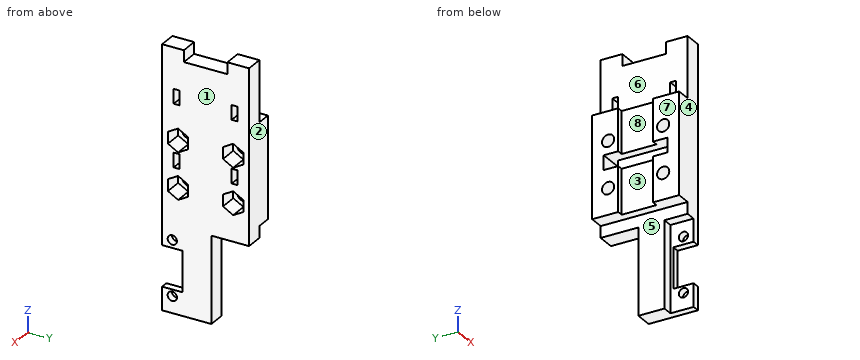
```python
from build123d import *

# Parameters (mm, degrees)
BOSS_EXTRUDE1_DEPTH = 30
CUT_EXTRUDE1_REACH  = 53.981
SKETCH2_R           = 2.1
CUT_EXTRUDE2_DEPTH  = 6
SKETCH4_W           = 5
SKETCH4_H           = 2
CUT_EXTRUDE3_DEPTH  = 52.980765673
SKETCH5_W           = 5
SKETCH5_H           = 18
CUT_EXTRUDE4_DEPTH  = 5
SKETCH6_W           = 4
SKETCH6_H           = 15
CUT_EXTRUDE5_DEPTH  = 52.15662225
BOSS_EXTRUDE2_DEPTH = 5
SKETCH7_W           = 2
SKETCH7_H           = 12
CUT_EXTRUDE6_DEPTH  = 51.418250664
LPATTERN1_COUNT     = 2
LPATTERN1_PITCH     = 16
BOSS_EXTRUDE3_DEPTH = 2.5
SKETCH10_W          = 29.8
SKETCH10_H          = 9
BOSS_EXTRUDE4_DEPTH = 3.5
SKETCH11_R          = 1.6
CUT_EXTRUDE7_DEPTH  = 59.330438023


with BuildPart() as part:
    # Sketch1 → Boss-Extrude1 (new body)
    with BuildSketch(Plane(origin=(0, 0, 0), x_dir=(1, 0, 0), z_dir=(0, 1, 0))):
        Polygon((0, 0), (5, 0), (5, 19), (11, 19), (11, -41), (5, -41), (5, -20), (0, -20), align=None)
    extrude(amount=BOSS_EXTRUDE1_DEPTH)

    # Sketch2 → Cut-Extrude1 (cut, up to next)
    with BuildSketch(Plane(origin=(11, 0, 0), x_dir=(0, 0, -1), z_dir=(1, 0, 0)), mode=Mode.PRIVATE) as cut_extrude1_sk1:
        with Locations((-10, 24.5)):
            Circle(SKETCH2_R)
    cut_extrude1_tool1 = extrude(cut_extrude1_sk1.sketch, amount=-CUT_EXTRUDE1_REACH, mode=Mode.PRIVATE) & part.part
    # Sketch2 → Cut-Extrude1 (cut, up to next)
    with BuildSketch(Plane(origin=(11, 0, 0), x_dir=(0, 0, -1), z_dir=(1, 0, 0)), mode=Mode.PRIVATE) as cut_extrude1_sk2:
        with Locations((-10, 5.5)):
            Circle(SKETCH2_R)
    cut_extrude1_tool2 = extrude(cut_extrude1_sk2.sketch, amount=-CUT_EXTRUDE1_REACH, mode=Mode.PRIVATE) & part.part
    cut_extrude1_1 = cut_extrude1_tool1.solids().sort_by_distance((11, 24.5, 10))[0]
    add(cut_extrude1_1, mode=Mode.SUBTRACT)
    cut_extrude1_2 = cut_extrude1_tool2.solids().sort_by_distance((11, 5.5, 10))[0]
    add(cut_extrude1_2, mode=Mode.SUBTRACT)
    cut_extrude1 = cut_extrude1_1 + cut_extrude1_2  # Cut-Extrude1 as one shape, for the pattern or mirror that repeats it

    # Sketch3 → Cut-Extrude2 (cut)
    with BuildSketch(Plane(origin=(11, 0, 0), x_dir=(0, 0, -1), z_dir=(1, 0, 0))):
        Polygon((-14.041451884, 24.5), (-12.020725942, 21), (-7.979274058, 21), (-5.958548116, 24.5), (-7.979274058, 28), (-12.020725942, 28), align=None)
        Polygon((-14.041451884, 5.5), (-12.020725942, 2), (-7.979274058, 2), (-5.958548116, 5.5), (-7.979274058, 9), (-12.020725942, 9), align=None)
    cut_extrude2 = extrude(amount=-CUT_EXTRUDE2_DEPTH, mode=Mode.SUBTRACT)

    # Sketch4 → Cut-Extrude3 (cut, through all)
    with BuildSketch(Plane(origin=(11, 0, 0), x_dir=(0, 0, -1), z_dir=(1, 0, 0))):
        with Locations((-24.5, 25)):
            Rectangle(SKETCH4_W, SKETCH4_H)
        with Locations((-24.5, 5)):
            Rectangle(SKETCH4_W, SKETCH4_H)
        with Locations((-3, 25)):
            Rectangle(SKETCH4_W, SKETCH4_H)
        with Locations((-3, 5)):
            Rectangle(SKETCH4_W, SKETCH4_H)
    extrude(amount=-CUT_EXTRUDE3_DEPTH, mode=Mode.SUBTRACT)

    # Sketch5 → Cut-Extrude4 (cut)
    with BuildSketch(Plane.ZY):
        with Locations((3, 15)):
            Rectangle(SKETCH5_W, SKETCH5_H)
    extrude(amount=-CUT_EXTRUDE4_DEPTH, mode=Mode.SUBTRACT)

    # Sketch6 → Cut-Extrude5 (cut, through all)
    with BuildSketch(Plane.ZY.offset(-5)):
        with Locations((39, 15)):
            Rectangle(SKETCH6_W, SKETCH6_H)
    extrude(amount=-CUT_EXTRUDE5_DEPTH, mode=Mode.SUBTRACT)

    # Sketch8 → Boss-Extrude2 (add)
    with BuildSketch(Plane.ZY.offset(-5)):
        Polygon((0, 30), (0, 14.791308029), (0, 0), (-15, 0), (-15, 30), align=None)
    extrude(amount=BOSS_EXTRUDE2_DEPTH)

    # Sketch7 → Cut-Extrude6 (cut, through all)
    with BuildSketch(Plane.XY.offset(20)):
        with Locations((1, 15)):
            Rectangle(SKETCH7_W, SKETCH7_H)
    extrude(amount=-CUT_EXTRUDE6_DEPTH, mode=Mode.SUBTRACT)

    # LPattern1: Cut-Extrude1, Cut-Extrude2 ×2
    with Locations(*[(0, 0, -i * LPATTERN1_PITCH) for i in range(1, LPATTERN1_COUNT)]):
        add(cut_extrude1, mode=Mode.SUBTRACT)
        add(cut_extrude2, mode=Mode.SUBTRACT)

    # Sketch9 → Boss-Extrude3 (add)
    with BuildSketch(Plane(origin=(11, 0, 0), x_dir=(0, 0, -1), z_dir=(1, 0, 0))):
        Polygon((19, 0), (26.8, 0), (26.8, 7), (40.8, 7), (40.8, 0), (48.8, 0), (48.8, 17), (19, 17), align=None)
    extrude(amount=-BOSS_EXTRUDE3_DEPTH)

    # Sketch10 → Boss-Extrude4 (add)
    with BuildSketch(Plane.ZY.offset(-8.5)):
        with Locations((-33.9, 12.5)):
            Rectangle(SKETCH10_W, SKETCH10_H)
    extrude(amount=BOSS_EXTRUDE4_DEPTH)

    # Sketch11 → Cut-Extrude7 (cut, through all)
    with BuildSketch(Plane(origin=(11, 0, 0), x_dir=(0, 0, -1), z_dir=(1, 0, 0))):
        with Locations((43.1, 3.5)):
            Circle(SKETCH11_R)
        with Locations((24.1, 3.5)):
            Circle(SKETCH11_R)
    extrude(amount=-CUT_EXTRUDE7_DEPTH, mode=Mode.SUBTRACT)


solid = part.part
```
Geometry: final body of the model. Coordinates: model frame, mm. Face numbers are marked on the shaded views. A direction names the side the tool comes from. Round coordinates to 2 decimals unless told otherwise and drop trailing zeros. Write each loop counter-clockwise with the first axis right and the second up, starting at its lowest first coordinate (ties: lowest second). Pieces come first, ordered by that corner, then holes. Notation, with made-up numbers: M 44.5,25 L 62.5,25 A29 cw 62.5,62 Z; hole C -9,-10 d7. An arc over 180 degrees is marked long. Answer in a Markdown table with one row per item. Add a question column.
(1) Cut plane C-C, the plane y = 14.25. Return the cut outline in (x, z), then the cut area to 3 significant figures.
(2) Draft query along Y for the marked faces 1, 2 and 3. Return one class per face: pulls with the +Y half, pulls with the -Y half, needs draft (parallel to the pull), parting line crosses it, or undercut.
(3) Cut plane B-B, the plane z = -43.1. Return the cut outline in (x, y).
(4) Cut plane D-D, the plane z = -6. Return the cut outline in (x, y), then the cut area to 3 significant figures.
(5) Reachability of the marked faces 4, 5, 6, 7 and 8 from +Z, -Z, +X, -X, +Y, -Y: full face, straight path, thin tool, end or side. Return the list, or none.
(6) Cut plane A-A, the plane z = 26. Return the cut outline in (x, y).
(7) Ray query, L1, parallel to Z at x = 3.75, y = 25; L2, parallel to Y at x = 1.15, z = -6; L3, parallel to Y at x = 3.35, z = -6. Return the intervals inside material, ascending.
(8) Contact query for flat-ended pins moving along their axis: pin 1 (5.5 mm diameter, centred on y = 5.5, z = 10, fed in from +X); pin 2 (2 mm diameter, centred on x = 7, y = 5, fed in from -Z); pin 3 (5 mm diameter, centred on y = 13.5, z = -29.5, fed in from -X). Output: stop coordinate, or through.
Established:
| question | item | result |
|---|---|---|
| 1 | outline | M 2,-15 L 5,-15 L 5,-48.8 L 11,-48.8 L 11,37 L 5,37 L 5,20 L 2,20 L 2,5.5 L 5,5.5 L 5,0.5 L 2,0.5 Z |
| 1 | area | 605 mm² |
| 2 | face 1 | needs draft |
| 2 | face 2 | pulls with the +Y half |
| 2 | face 3 | undercut |
| 3 | outline | M 5,8 L 8.5,8 L 8.5,5.1 L 11,5.1 L 11,17 L 5,17 Z; M 8.5,0 L 11,0 L 11,1.9 L 8.5,1.9 Z |
| 4 | outline | M 0,0 L 11,0 L 11,2 L 5,2 L 5,3.4 L 0,3.4 Z; M 0,7.6 L 5,7.6 L 5,9 L 11,9 L 11,21 L 5,21 L 5,22.4 L 0,22.4 L 0,21 L 2,21 L 2,9 L 0,9 Z; M 0,26.6 L 5,26.6 L 5,28 L 11,28 L 11,30 L 0,30 Z |
| 4 | area | 180 mm² |
| 5 | face 4 | +Z, -Z, +X, -X, -Y |
| 5 | face 5 | -Z, -X, +Y, -Y |
| 5 | face 6 | +Z, -X, +Y, -Y |
| 5 | face 7 | +Z, -Z, -X, +Y, -Y |
| 5 | face 8 | +Z, -Z, -X |
| 6 | outline | M 5,0 L 11,0 L 11,4 L 5,4 Z; M 5,6 L 11,6 L 11,24 L 5,24 Z; M 5,26 L 11,26 L 11,30 L 5,30 Z |
| 7 | L1 | -15 to -8.04, -3.96 to 0.5, 5.5 to 7.96, 12.04 to 20 |
| 7 | L2 | 0 to 3.4, 7.6 to 9, 21 to 22.4, 26.6 to 30 |
| 7 | L3 | 0 to 3.4, 7.6 to 22.4, 26.6 to 30 |
| 8 | pin 1 | x = 5 |
| 8 | pin 2 | z = -19 |
| 8 | pin 3 | x = 5 |
